```python
from build123d import *

# Parameters (mm, degrees)
SKETCH1_R           = 4.95
BOSS_EXTRUDE1_DEPTH = 7.3
CHAMFER1_SIZE       = 0.5
CHAMFER1_SIZE2      = 0.4
SKETCH2_R           = 0.32
BOSS_EXTRUDE2_DEPTH = 10
SKETCH3_R           = 4.45
CUT_EXTRUDE1_DEPTH  = 0.1


with BuildPart() as part:
    # Sketch1 → Boss-Extrude1 (new body)
    with BuildSketch(Plane(origin=(0, 0, 0), x_dir=(1, 0, 0), z_dir=(0, 1, 0))):
        Circle(SKETCH1_R)
    extrude(amount=BOSS_EXTRUDE1_DEPTH)

    # Chamfer1
    chamfer1_edges = [part.edges().sort_by_distance(p)[0] for p in [
        (-4.95, 7.3, 0),
    ]]
    chamfer1_side = [part.faces().sort_by_distance(p)[0] for p in [
        (-4.95, 3.65, 0),
    ]]
    chamfer(chamfer1_edges, length=CHAMFER1_SIZE, length2=CHAMFER1_SIZE2, reference=chamfer1_side[0])

    # Sketch2 → Boss-Extrude2 (add)
    with BuildSketch(Plane.XZ):
        with Locations((-2.5, 0)):
            Circle(SKETCH2_R)
        with Locations((2.5, 0)):
            Circle(SKETCH2_R)
    extrude(amount=BOSS_EXTRUDE2_DEPTH)

    # Sketch3 → Cut-Extrude1 (cut)
    with BuildSketch(Plane(origin=(0, 7.3, 0), x_dir=(1, 0, 0), z_dir=(0, 1, 0))):
        Circle(SKETCH3_R)
    extrude(amount=-CUT_EXTRUDE1_DEPTH, mode=Mode.SUBTRACT)


solid = part.part
```
Geometry check sheet. Reference: the model listing, model coordinates, mm. Coordinates: 2 decimals unless noted, no trailing zeros. Order: outer loops, then holes, each group sorted by start corner. A loop starts at its lowest first (then second) coordinate and runs counter-clockwise, first axis right, second up. Notation, with made-up numbers: M 52.5,-2.5 L 85.5,-2.5 A14 ccw 85.5,23.5 Z; hole C 28.5,-19.5 d10. An arc over 180 degrees is marked long. One line per question, with ' | ' between items. Start each with the question number.
Item 1: Material ranges on L1, parallel to Y at x = -0.25, z = 0.75; L2, parallel to X at y = 6.75, z = 0.25; L3, parallel to X at y = 1.25, z = -4, recorded low to high. Write a range as [from, to].
Item 2: Cross-section at A-A on z = 0. Enter the section's corners in (x, y).
Item 3: Draft check along Z on faces 1 (the flat face through (0, 0, 0)), 2 (the cylindrical face through (4.72, 3.35, -1.49)), 3 (the flat face through (0, 7.2, 0)). Enter one of: pulls with the +Z half, pulls with the -Z half, needs draft (parallel to the pull), parting line crosses it, or undercut.
Item 4: Cross-section at C-C on y = -8.25. Enter the section's corners in (x, z).
Item 5: Cross-section at B-B on x = 0. Enter the section's corners in (y, z), then the cut area to 3 significant figures.
Item 6: Cross-section at D-D on y = 2.75. Enter the section's corners in (x, z).
Item 7: Gauge pin test, flat ends, axial feed: pin 1 (5 mm diameter, centred on x = -4, y = -7.5, fed in from -Z); pin 2 (2.5 mm diameter, centred on x = -1, z = 0.5, fed in from +Y); pin 3 (1.5 mm diameter, centred on y = 3, z = 3, fed in from -X). Record the tip position at first contact, or that the pin passes through.
Findings:
1) L1: y = [0, 7.2] | L2: x = [-4.94, 4.94] | L3: x = [-2.92, 2.92]
2) outline: M -4.95,0 L -2.82,0 L -2.82,-10 L -2.18,-10 L -2.18,0 L 2.18,0 L 2.18,-10 L 2.82,-10 L 2.82,0 L 4.95,0 L 4.95,6.8 L 4.55,7.3 L 4.45,7.3 L 4.45,7.2 L -4.45,7.2 L -4.45,7.3 L -4.55,7.3 L -4.95,6.8 Z
3) face 1: needs draft | face 2: parting line crosses it | face 3: undercut
4) outline: C -2.5,0 d0.64; C 2.5,0 d0.64
5) outline: M 0,-4.95 L 6.8,-4.95 L 7.3,-4.55 L 7.3,-4.45 L 7.2,-4.45 L 7.2,4.45 L 7.3,4.45 L 7.3,4.55 L 6.8,4.95 L 0,4.95 Z | area: 71.2 mm²
6) outline: C 0,0 d9.9
7) pin 1: stops at z = -0.32 | pin 2: stops at y = 7.2 | pin 3: stops at x = -4.41
